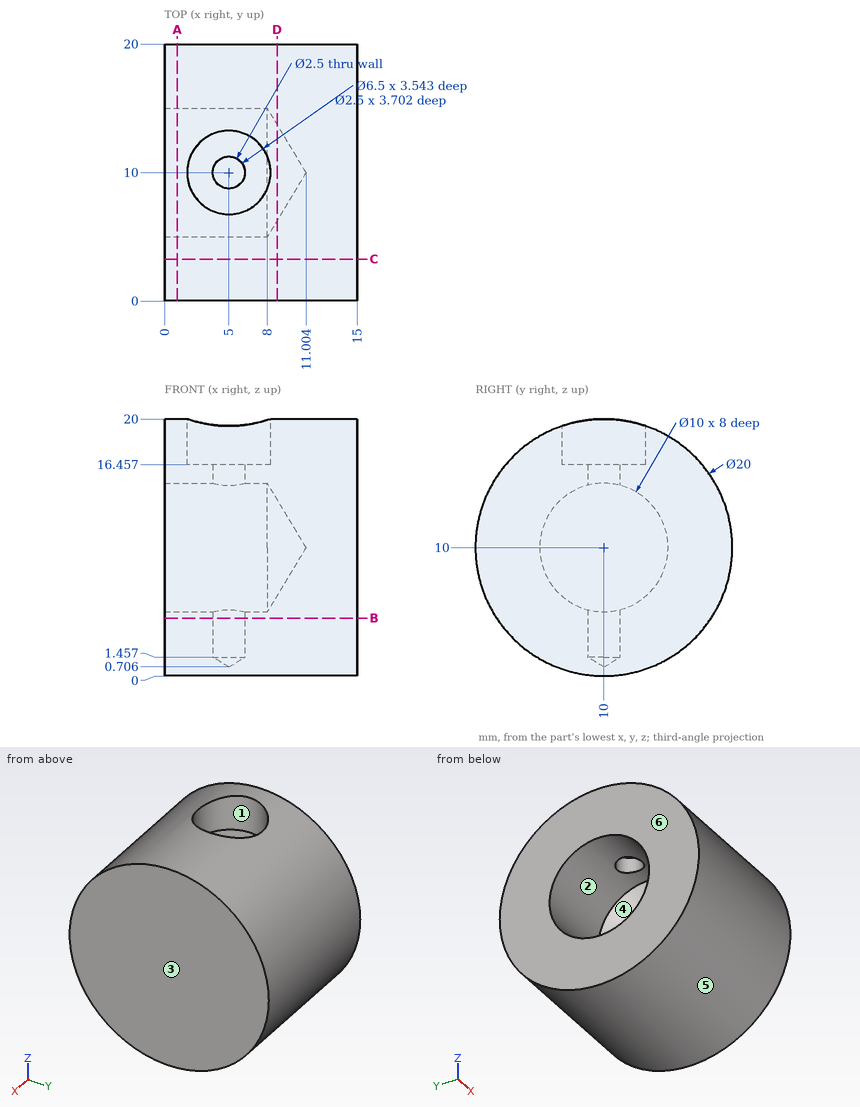
Part print with two shaded views. Sizes in mm from the minimum x, y, z corner. A direction names the side the tool comes from. Round coordinates to 2 decimals unless told otherwise and drop trailing zeros. Loops run counter-clockwise (first coordinate to the right, second up) from the corner with the lowest first, then second, coordinate; pieces in that order, holes last.
Item 1: Pin check, flat tips, straight feed: P1, Ø4, axis at x = 5, y = 10, coming from the +Z side; P2, Ø1, axis at x = 7.5, z = 6, coming from the +Y side; P3, Ø5, axis at x = 4.5, y = 4.5, coming from the +Z side. Stop position of each tip, or through.
Item 2: Saw through at C-C (y = 3.25). List the corners of the cut face in (x, z).
Item 3: Drill centre lines: line 1 along Z through (x, y) = (6.75, 9.75); line 2 along Y through (x, z) = (0.5, 6) (1 decimal); line 3 along Y through (x, z) = (2, 12). Where is each one in solid material? Low to high.
Item 4: Saw through at A-A (x = 1). List the corners of the cut face in (y, z).
Item 5: Saw through at B-B (z = 4.5). List the corners of the cut face in (x, y).
Item 6: Which spindle directions (+Z, -Z, +X, -X, +Y, -Y) get a long thin tool onto all of the face, cutting with end or side? Do the marked faces 1, 2 and 3. Say none if no direction does.
Item 7: Saw through at D-D (x = 8.75). List the corners of the cut face in (y, z).
Item 8: Two-plate mould, pull along Z, no slides. Class the marked faces 4, 5 and 6: released by +Z, released by -Z, zero draft, split by the parting line, or undercut.
Worked answers:
1. P1: stops at z = 16.46
1. P2: stops at y = 19.37
1. P3: stops at z = 19.52
2. outline: (0, 2.62) - (15, 2.62) - (15, 17.38) - (0, 17.38) - close
3. line 1: z = 0 to 5.01, 14.99 to 16.46
3. line 2: y = 0.8 to 7, 13 to 19.2
3. line 3: y = 0.2 to 5.42, 14.58 to 19.8
4. outline: circle Ø20 at (10, 10); hole circle Ø10 at (10, 10)
5. outline: (0, 1.65) - (15, 1.65) - (15, 18.35) - (0, 18.35) - close; hole circle Ø2.5 at (5, 10)
6. face 1: +Z
6. face 2: -X
6. face 3: +Z, -Z, +X, +Y, -Y
7. outline: circle Ø20 at (10, 10); hole circle Ø7.5 at (10, 10)
8. face 4: undercut
8. face 5: split by the parting line
8. face 6: zero draft
